Read the model definition and answer for the solid it produces. Units are mm, in the model's axes. A direction names the side the tool comes from. Round coordinates to 2 decimals unless told otherwise and drop trailing zeros. Order: outer loops, then holes, each group sorted by start corner. A loop starts at its lowest first (then second) coordinate and runs counter-clockwise, first axis right, second up. Notation, with made-up numbers: (29, 27) - (85, 27) arc R27 ccw to (85, 49) - close; hole circle Ø4 at (4, 9.5). An arc over 180 degrees is marked (long way). Answer as a JSON object with one key per item and string values. Group by question number.
Q1. A cutting plane is placed at C-C on z = 4. Determine the outline of the cut face in (x, y), and give its area (3 significant figures).
Q2. A cutting plane is placed at D-D on x = 49. Determine the outline of the cut face in (y, z).
Q3. A cutting plane is placed at A-A on y = -17.5. Determine the outline of the cut face in (x, z), and give its area (3 significant figures).
Q4. Consider line 1 (X direction, y = -63.5, z = 9.5); line 2 (X direction, y = -75.5, z = 14); line 3 (Y direction, x = 48.5, z = 11.5). Determine where each line is inside the solid, lowest interval first.
Q5. A cutting plane is placed at B-B on x = 8. Determine the outline of the cut face in (y, z), and give its area (3 significant figures).
Q6. A tool of negligible diameter and unlimited length cuts with its end or side. For faces 1 (the flat face through (6, -87.394, 6)), 2 (the cylindrical face through (34.413, -11.189, 11.437)), from which of +Z, -Z, +X, -X, +Y, -Y can it reach the whole face along a straight path? Write none if from no direction.
Q7. Given pin 1 Ø3 at (y, z) = (-26, 1.5) entering from +X; pin 2 Ø6 at (y, z) = (-76.5, 12.5) entering from +X; pin 3 Ø10 at (x, y) = (10, -12) entering from +Z, each flat-ended and moving along its own axis, determine where each tip first touches the part or whether it passes through.
```python
from build123d import *

# Parameters (mm, degrees)
F1_DEPTH = 87.394075
F3_DEPTH = 56.96498


with BuildPart() as f1:
    # F0 (on Front) → F1 (new body)
    with BuildSketch(Plane.XZ):
        with BuildLine():
            ThreePointArc((16, 0), (11.313708, 11.313708), (0, 16))
            Line((0, 16), (0, 0))
            Line((0, 0), (16, 0))
        make_face()
    extrude(amount=F1_DEPTH)

    # F2 (on Right) → F3 (join)
    with BuildSketch(Plane.YZ):
        with BuildLine():
            Line((-16, 0), (0, 0))
            Line((0, 0), (0, 16))
            ThreePointArc((0, 16), (-11.313708, 11.313708), (-16, 0))
        make_face()
    extrude(amount=F3_DEPTH)


solid = f1.part
```
Result set:
{
 "1": {"outline": "(0, -87.39) - (15.49, -87.39) - (15.49, -15.49) - (56.96, -15.49) - (56.96, 0) - (0, 0) - close", "area": "2,000 mm²"},
 "2": {"outline": "(-16, 0) - (0, 0) - (0, 16) arc R16 ccw to start"},
 "3": {"outline": "(0, 0) - (16, 0) arc R16 ccw to (0, 16) - close", "area": "201 mm²"},
 "4": {"line 1": "x = 0 to 12.87", "line 2": "x = 0 to 7.75", "line 3": "y = -11.12 to 0"},
 "5": {"outline": "(-87.39, 0) - (0, 0) - (0, 16) arc R16 ccw to (-8, 13.86) - (-87.39, 13.86) - close", "area": "1,220 mm²"},
 "6": {"face 1": "+Z, -Z, +X, -X, -Y", "face 2": "+Z, +X, -Y"},
 "7": {"pin 1": "stops at x = 16", "pin 2": "stops at x = 12.87", "pin 3": "stops at z = 15.2"}
}
